from build123d import *

# Parameters (mm, degrees)
SKETCH1_R                   = 9.525
BOSS_EXTRUDE1_DEPTH         = 342.9
SKETCH2_R                   = 6.35
BOSS_EXTRUDE2_DEPTH         = 9.779
F_1_4_20_TAPPED_HOLE1_D     = 5.1054
F_1_4_20_TAPPED_HOLE1_DEPTH = 25.4
F_1_4_20_TAPPED_HOLE1_TIP   = 1.533816902
BOSS_EXTRUDE3_START         = 9.779
SKETCH5_R                   = 6.35
BOSS_EXTRUDE3_DEPTH         = 9.779
F_1_4_20_TAPPED_HOLE2_D     = 5.1054
F_1_4_20_TAPPED_HOLE2_DEPTH = 25.4
F_1_4_20_TAPPED_HOLE2_TIP   = 1.533816902


with BuildPart() as part:
    # Sketch1 → Boss-Extrude1 (new body)
    with BuildSketch(Plane.XY):
        Circle(SKETCH1_R)
    extrude(amount=BOSS_EXTRUDE1_DEPTH)

    # Sketch2 → Boss-Extrude2 (add)
    with BuildSketch(Plane.XY.offset(342.9)):
        Circle(SKETCH2_R)
    extrude(amount=BOSS_EXTRUDE2_DEPTH)

    # 1/4-20 Tapped Hole1
    with Locations(Plane.XY.offset(352.679)):
        with Locations((0, 0)):
            Hole(F_1_4_20_TAPPED_HOLE1_D / 2, depth=F_1_4_20_TAPPED_HOLE1_DEPTH)
            with Locations((0, 0, -(F_1_4_20_TAPPED_HOLE1_DEPTH + F_1_4_20_TAPPED_HOLE1_TIP / 2))):  # 118° drill point
                Cone(0, F_1_4_20_TAPPED_HOLE1_D / 2, F_1_4_20_TAPPED_HOLE1_TIP, mode=Mode.SUBTRACT)

    # Sketch5 → Boss-Extrude3 (add)
    with BuildSketch(Plane(origin=(0, 0, 0), x_dir=(-1, 0, 0), z_dir=(0, 0, -1)).offset(BOSS_EXTRUDE3_START)):
        with Locations(Location((0, 0, 0), (0, 0, 180))):
            Circle(SKETCH5_R)
    extrude(amount=-BOSS_EXTRUDE3_DEPTH)

    # 1/4-20 Tapped Hole2
    with Locations(Plane(origin=(0, 0, -9.779), x_dir=(-1, 0, 0), z_dir=(0, 0, -1))):
        with Locations((0, 0)):
            Hole(F_1_4_20_TAPPED_HOLE2_D / 2, depth=F_1_4_20_TAPPED_HOLE2_DEPTH)
            with Locations((0, 0, -(F_1_4_20_TAPPED_HOLE2_DEPTH + F_1_4_20_TAPPED_HOLE2_TIP / 2))):  # 118° drill point
                Cone(0, F_1_4_20_TAPPED_HOLE2_D / 2, F_1_4_20_TAPPED_HOLE2_TIP, mode=Mode.SUBTRACT)


solid = part.part
Can you work these out from the model? Positions are in its coordinate system, mm. A direction names the side the tool comes from. Give positions to 0.01 mm unless a question says otherwise; leave off trailing zeros. Order: outer loops, then holes, each group sorted by start corner. A loop starts at its lowest first (then second) coordinate and runs counter-clockwise, first axis right, second up. Notation, with made-up numbers: M 55,-35.5 L 112,-35.5 A27 cw 112,-10.5 Z; hole C 1.5,36.25 d2. An arc over 180 degrees is marked long. One line per item, written item: value.
Item 1: For pin 1 (4.5 mm diameter, centred on x = 0, y = 0, fed in from +Z); pin 2 (6 mm diameter, centred on y = 7.5, z = 157, fed in from -X) (3 decimals); pin 3 (6.5 mm diameter, centred on x = 0, y = 0, fed in from -Z); pin 4 (4 mm diameter, centred on x = -7, y = 6.5, fed in from -Z), each with a flat end and sliding along its axis, tell me the tip position at first contact or that it passes through.
Verdict:
pin 1: z = 327.1
pin 2: x = -8.395
pin 3: z = -9.78
pin 4: z = 0
Item 2: For faces 1 (the face through (-1.38, -6.2, 347.72)), 2 (the face through (-7.559, -5.796, 169.05)), 3 (the face through (2, -6.2, 0)), which set-ups out of +Z, -Z, +X, -X, +Y, -Y let a thin tool reach every point of the face, with its end or its side?
Verdict:
face 1: +Z
face 2: +Z, -Z
face 3: -Z
Item 3: If we section it at A-A on z = 233: Write out the boundary of the cut face in (x, y) (3 decimals).
Verdict:
outline: C 0,0 d19.05
Item 4: Please list where these lines run through material, in increasing order: line 1 (Y direction, x = 0, z = 339.25) (3 decimals); line 2 (Z direction, x = -8.5, y = 4); line 3 (Y direction, x = 0, z = 344).
Verdict:
line 1: -9.525 to -2.553, 2.553 to 9.525
line 2: 0 to 342.9
line 3: -6.35 to -2.55, 2.55 to 6.35
